Check sheet for the modelled part. Datum: model origin and axes. Units: mm. Face numbers are marked on the shaded views. Give positions to 0.01 mm unless a question says otherwise; leave off trailing zeros. Order: outer loops, then holes, each group sorted by start corner. A loop starts at its lowest first (then second) coordinate and runs counter-clockwise, first axis right, second up.
Item 1: Gauge pin test, flat ends, axial feed: P1, Ø1.5, axis at x = -21.5, z = -25, coming from the +Y side; P2, Ø1.6, axis at x = -35, y = -2.5, coming from the +Z side; P3, Ø1, axis at x = -36, y = -1.5, coming from the -Z side; P4, Ø3, axis at x = -43.5, z = -21.5, coming from the +Y side. Record the tip position at first contact, or that the pin passes through.
Item 2: Release check for a two-part mould opening along Y. For the marked faces 1 and 2 record: released by +Y, released by -Y, zero draft, split by the parting line, or undercut.
Item 3: Material ranges on line 1 along Z through (x, y) = (-50.5, -1.65); line 2 along X through (y, z) = (-0.6, -7); line 3 along Z through (x, y) = (-40.5, -2.6), recorded low to high.
Item 4: Sectioned sample at B-B on z = -12. Record the boundary of the cut face in (x, y) (3 decimals), and give its area (3 significant figures).
Item 5: Sectioned sample at C-C on y = -2.5. Record the boundary of the cut face in (x, z), and give its area (3 significant figures).
Item 6: Sectioned sample at A-A on x = -28.5. Record the boundary of the cut face in (y, z) (3 decimals).
from build123d import *

# Parameters (mm, degrees)
F0_W     = 41.142106
F0_H     = 20.32
F1_DEPTH = 3.175


with BuildPart() as f1:
    # F0 (on Front) → F1 (new body)
    with BuildSketch(Plane.XZ):
        Polygon((-50.709821, 13.180559), (-60.869821, 13.180559), (-60.869821, -37.619441), (-50.709821, -37.619441), (-50.709821, -40.794441), (-40.549821, -40.794441), (-40.549821, -37.619441), (-25.309821, -37.619441), (-25.309821, -40.794441), (-15.149821, -40.794441), (-15.149821, -37.619441), (-4.989821, -37.619441), (-4.989821, 13.180559), (-15.149821, 13.180559), (-15.149821, 16.355559), (-25.309821, 16.355559), (-25.309821, 13.180559), (-40.549821, 13.180559), (-40.549821, 16.355559), (-50.709821, 16.355559), align=None)
        with Locations((-32.580219, -14.759441)):
            Rectangle(F0_W, F0_H, mode=Mode.SUBTRACT)
    extrude(amount=F1_DEPTH)


solid = f1.part
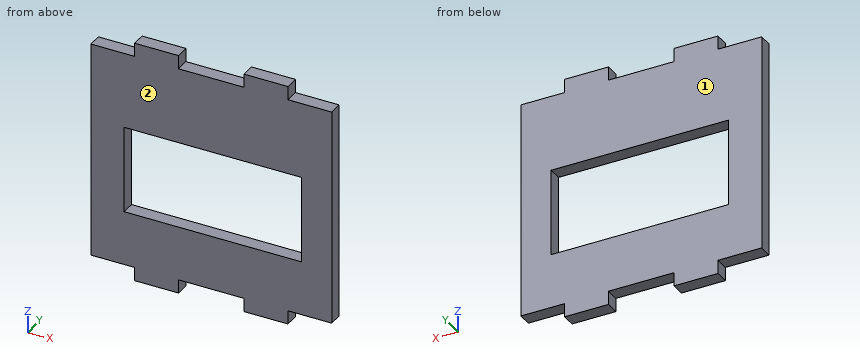
Report:
1. P1: stops at y = 0
1. P2: stops at z = 13.18
1. P3: stops at z = -37.62
1. P4: passes through
2. face 1: released by +Y
2. face 2: released by -Y
3. line 1: z = -40.79 to -24.92, -4.6 to 16.36
3. line 2: x = -60.87 to -53.15, -12.01 to -4.99
3. line 3: z = -37.62 to -24.92, -4.6 to 13.18
4. outline: (-60.87, -3.175) - (-53.151, -3.175) - (-53.151, 0) - (-60.87, 0) - close; (-12.009, -3.175) - (-4.99, -3.175) - (-4.99, 0) - (-12.009, 0) - close
4. area: 46.8 mm2
5. outline: (-60.87, -37.62) - (-50.71, -37.62) - (-50.71, -40.79) - (-40.55, -40.79) - (-40.55, -37.62) - (-25.31, -37.62) - (-25.31, -40.79) - (-15.15, -40.79) - (-15.15, -37.62) - (-4.99, -37.62) - (-4.99, 13.18) - (-15.15, 13.18) - (-15.15, 16.36) - (-25.31, 16.36) - (-25.31, 13.18) - (-40.55, 13.18) - (-40.55, 16.36) - (-50.71, 16.36) - (-50.71, 13.18) - (-60.87, 13.18) - close; hole (-53.15, -24.92) - (-12.01, -24.92) - (-12.01, -4.6) - (-53.15, -4.6) - close
5. area: 2,130 mm2
6. outline: (-3.175, -37.619) - (0, -37.619) - (0, -24.919) - (-3.175, -24.919) - close; (-3.175, -4.599) - (0, -4.599) - (0, 13.181) - (-3.175, 13.181) - close
